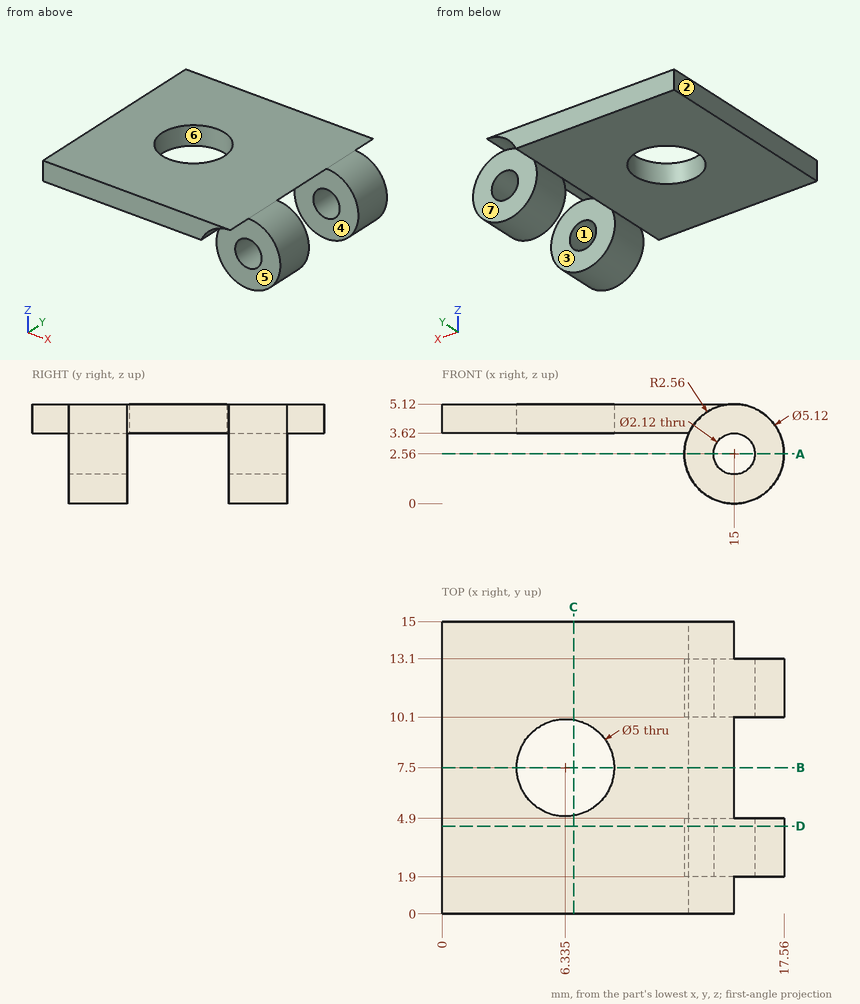
The drawing under review shows one solid part. Ordinate dimensions are in mm from its lowest x, y, z. A direction names the side the tool comes from. Coordinates: 2 decimals unless noted, no trailing zeros. Order: outer loops, then holes, each group sorted by start corner. A loop starts at its lowest first (then second) coordinate and runs counter-clockwise, first axis right, second up. Notation, with made-up numbers: (-6, 40.5) -> (29, 40.5) arc R24 cw to (29, 61.5) -> close; hole circle Ø4 at (-17, 22.5). An arc over 180 degrees is marked (long way). Answer in a Markdown table with one row per item. Add a question column.
Item 1: We need section C-C on x = 6.75. Write out the cut boundary in (y, z), plus the area to 3 significant figures.
Item 2: We need section A-A on z = 2.56. Write out the cut boundary in (x, y), plus the area to 3 significant figures.
Item 3: Clearance check with flat-ended pins moving along their axes: pin 1 (2.5 mm diameter, centred on x = 15.5, z = 2, fed in from +Y); pin 2 (1.3 mm diameter, centred on x = 15, z = 2.56, fed in from -Y); pin 3 (1.5 mm diameter, centred on y = 5.5, z = 1, fed in from +X). State where each tip first meets the part, or that it passes through.
Item 4: Mouldability with a two-part tool opening along X and no side actions: class the marked faces 1, 2 and 3 as +X half, -X half, draft (parallel to the pull), parting line (faces both ways), or undercut.
Item 5: To check wall thickness, follow probe 1 along Y at (x, z) = (14.5, 4.5); probe 2 along X at (y, z) = (11.9, 2.56); probe 3 along Z at (x, y) = (11, 2.75). State the ranges of each line that lie inside material, in increasing order.
Item 6: Machinability: for the marked faces 4, 5, 6 and 7, which of the approach directions +Z, -Z, +X, -X, +Y, -Y give a long, thin tool a straight path to every point of the face, cutting with its end or side? Answer none if there is none.
Item 7: We need section D-D on y = 4.5. Write out the cut boundary in (x, z).
Item 8: We need section B-B on y = 7.5. Write out the cut boundary in (x, z) (3 decimals), plus the area to 3 significant figures.
Final values:
| question | item | result |
|---|---|---|
| 1 | outline | (0, 3.62) -> (5.03, 3.62) -> (5.03, 5.12) -> (0, 5.12) -> close; (9.97, 3.62) -> (15, 3.62) -> (15, 5.12) -> (9.97, 5.12) -> close |
| 1 | area | 15.1 mm2 |
| 2 | outline | (12.44, 1.9) -> (13.94, 1.9) -> (13.94, 4.9) -> (12.44, 4.9) -> close; (12.44, 10.1) -> (13.94, 10.1) -> (13.94, 13.1) -> (12.44, 13.1) -> close; (16.06, 1.9) -> (17.56, 1.9) -> (17.56, 4.9) -> (16.06, 4.9) -> close; (16.06, 10.1) -> (17.56, 10.1) -> (17.56, 13.1) -> (16.06, 13.1) -> close |
| 2 | area | 18.0 mm2 |
| 3 | pin 1 | stops at y = 13.1 |
| 3 | pin 2 | passes through |
| 3 | pin 3 | stops at x = 17.31 |
| 4 | face 1 | undercut |
| 4 | face 2 | -X half |
| 4 | face 3 | draft |
| 5 | probe 1 | y = 1.9 to 4.9, 10.1 to 13.1 |
| 5 | probe 2 | x = 12.44 to 13.94, 16.06 to 17.56 |
| 5 | probe 3 | z = 3.62 to 5.12 |
| 6 | face 4 | -Z, +X |
| 6 | face 5 | -Z, +X, -Y |
| 6 | face 6 | +Z, -Z |
| 6 | face 7 | -Z, +X, +Y |
| 7 | outline | (0, 3.62) -> (12.67, 3.62) arc R2.56 ccw (long way) to (15, 5.12) -> (0, 5.12) -> close; hole circle Ø2.12 at (15, 2.56) |
| 8 | outline | (0, 3.62) -> (3.835, 3.62) -> (3.835, 5.12) -> (0, 5.12) -> close; (8.835, 3.62) -> (12.67, 3.62) arc R2.56 cw to (15, 5.12) -> (8.835, 5.12) -> close |
| 8 | area | 12.5 mm2 |
